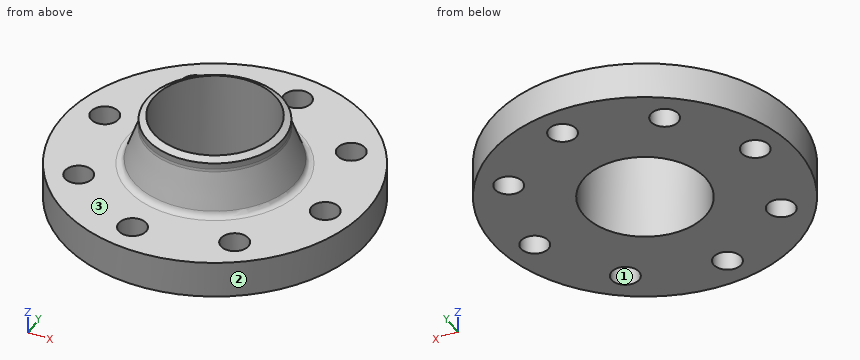
```python
from build123d import *

# Parameters (mm, degrees)
F2_R     = 9
F3_DEPTH = 25
F4_R     = 5


with BuildPart() as f1:
    # F0 (on Front) → F1 (revolve)
    with BuildSketch(Plane.XZ):
        Polygon((-100, 0), (-40, 0), (-40, 58), (-44.45, 55.430791), (-44.45, 50.430791), (-54.070021, 24), (-100, 24), align=None)
    revolve(axis=Axis((0, 0, 3.000721), (0, 0, -1)))

    # F2 (on face) → F3 (cut)
    with BuildSketch(Plane.XY.offset(24)):
        with Locations((-46.161917, 65.338177)):
            Circle(F2_R)
        with Locations((-78.842473, 13.559663)):
            Circle(F2_R)
        with Locations((-65.338177, -46.161917)):
            Circle(F2_R)
        with Locations((-13.559663, -78.842473)):
            Circle(F2_R)
        with Locations((46.161917, -65.338177)):
            Circle(F2_R)
        with Locations((78.842473, -13.559663)):
            Circle(F2_R)
        with Locations((65.338177, 46.161917)):
            Circle(F2_R)
        with Locations((13.559663, 78.842473)):
            Circle(F2_R)
    extrude(amount=-F3_DEPTH, mode=Mode.SUBTRACT)

    # F4
    f4_edges = [f1.edges().sort_by_distance(p)[0] for p in [
        (54.070021, 0, 24),
        (44.45, 0, 50.430791),
    ]]
    fillet(f4_edges, radius=F4_R)


solid = f1.part
```
Design review of the part built by this model. Coordinates are the model's own, in mm. Face numbers are marked on the shaded views. Round coordinates to 2 decimals unless told otherwise and drop trailing zeros. Write each loop counter-clockwise with the first axis right and the second up, starting at its lowest first coordinate (ties: lowest second). Pieces come first, ordered by that corner, then holes. Notation, with made-up numbers: (31.25, -0.75) -> (73.25, -0.75) arc R13 ccw to (73.25, 14.25) -> close; hole circle Ø9 at (77.5, -18). An arc over 180 degrees is marked (long way). Write item = value, one per line. Start each with the question number.
1) Take a section at B-B, the plane y = -82.5. State the section outline as (x, z) points.
2) Mouldability with a two-part tool opening along X and no side actions: class the marked faces 1, 2 and 3 as +X half, -X half, draft (parallel to the pull), parting line (faces both ways), or undercut.
3) Take a section at C-C, the plane z = 39. State the section outline as (x, y) points, plus the area to 3 significant figures.
4) Wall thickness on probe 1 along X at (y, z) = (6, 18); probe 2 along X at (y, z) = (-13.5, 19.5); probe 3 along X at (y, z) = (0.5, 21.5): over which ranges is each line inside the solid? List them lowest first. Write a range as from..to.
5) Clearance check with flat-ended pins moving along their axes: pin 1 (3 mm diameter, centred on y = -4.5, z = 23.5, fed in from -X) (3 decimals); pin 2 (8 mm diameter, centred on x = 49, z = 25.5, fed in from -Y); pin 3 (14.5 mm diameter, centred on x = -46.16, y = 65.34, fed in from +Z); pin 4 (2 mm diameter, centred on y = 39, z = 42, fed in from -X). State where each tip first meets the part, or that it passes through.
6) Take a section at A-A, the plane x = 66. State the section outline as (y, z) points, plus the area to 3 significant figures.
7) Take a section at D-D, the plane x = 13. Count the separate pieces of the cut face and the enclosed holes in it, plus the area to 3 significant figures.
Results list:
q1.outline = (-56.51, 0) -> (-21.78, 0) -> (-21.78, 24) -> (-56.51, 24) -> close; (-5.34, 0) -> (56.51, 0) -> (56.51, 24) -> (-5.34, 24) -> close
q2.face_1 = undercut
q2.face_2 = parting line
q2.face_3 = draft
q3.outline = circle Ø97.22 at (0, 0); hole circle Ø80 at (0, 0)
q3.area = 2,400 mm²
q4.probe_1 = -99.82..-83.73, -73.96..-39.55, 39.55..99.82
q4.probe_2 = -99.08..-37.65, 37.65..69.84, 87.84..99.08
q4.probe_3 = -100..-40, 40..100
q5.pin_1 = -99.955
q5.pin_2 = -89.16
q5.pin_3 = through
q5.pin_4 = -28.66
q6.outline = (-75.13, 0) -> (37.19, 0) -> (37.19, 24) -> (-75.13, 24) -> close; (55.14, 0) -> (75.13, 0) -> (75.13, 24) -> (55.14, 24) -> close
q6.area = 3,180 mm²
q7.separate_pieces = 3
q7.enclosed_holes = 0
q7.area = 3,090 mm²
